from build123d import *

# Parameters (mm, degrees)
F0_W     = 69.0372
F0_H     = 63.5
F1_DEPTH = 4.7625
F2_R     = 3.1877
F3_DEPTH = 4.7635
F4_R     = 2.54
F5_DEPTH = 4.7635
F4_R_2   = 7.527211353
F4_R_3   = 7.5272138977
F6_DEPTH = 0.508
F8_DEPTH = 69.0382


with BuildPart() as f1:
    # F0 (on Top) → F1 (new body)
    with BuildSketch(Plane.XY):
        with Locations((0, -31.75)):
            Rectangle(F0_W, F0_H)
    extrude(amount=F1_DEPTH)

    # F2 (on face) → F3 (cut, through all)
    with BuildSketch(Plane.XY.offset(4.7625)):
        with Locations((25.4, -53.975)):
            Circle(F2_R)
        with Locations((-25.4, -53.975)):
            Circle(F2_R)
    extrude(amount=-F3_DEPTH, mode=Mode.SUBTRACT)

    # F4 (on face) → F5 (cut, through all)
    with BuildSketch(Plane.XY.offset(4.7625)):
        with Locations((-19.05, -19.05)):
            Circle(F4_R)
        with Locations((19.05, -19.05)):
            Circle(F4_R)
    extrude(amount=-F5_DEPTH, mode=Mode.SUBTRACT)

    # F4 (on face) → F6 (cut)
    with BuildSketch(Plane.XY.offset(4.7625)):
        with Locations((-19.05, -19.05)):
            Circle(F4_R_2)
        with Locations((-19.05, -19.05)):
            Circle(F4_R, mode=Mode.SUBTRACT)
        with Locations((19.05, -19.05)):
            Circle(F4_R_3)
        with Locations((19.05, -19.05)):
            Circle(F4_R, mode=Mode.SUBTRACT)
    extrude(amount=-F6_DEPTH, mode=Mode.SUBTRACT)

    # F7 (on face) → F8 (cut, through all)
    with BuildSketch(Plane.YZ.offset(34.5186)):
        with BuildLine():
            ThreePointArc((-1.9939, 4.7625), (-1.5875, 4.3561), (-1.1811, 4.7625))
            Line((-1.1811, 4.7625), (-1.9939, 4.7625))
        make_face()
        with BuildLine():
            Line((-1.9939, 0), (-1.1811, 0))
            ThreePointArc((-1.1811, 0), (-1.5875, 0.4064), (-1.9939, 0))
        make_face()
    extrude(amount=-F8_DEPTH, mode=Mode.SUBTRACT)


solid = f1.part
Work out the finished part from the listing and answer in its coordinate system (mm). A direction names the side the tool comes from. Give positions to 0.01 mm unless a question says otherwise; leave off trailing zeros. Order: outer loops, then holes, each group sorted by start corner. A loop starts at its lowest first (then second) coordinate and runs counter-clockwise, first axis right, second up. Notation, with made-up numbers: (-25, 63.5) -> (7, 63.5) arc R35 cw to (7, 101.5) -> close; hole circle Ø2 at (31, -25). An arc over 180 degrees is marked (long way). One line per item, written item: value.
Item 1: Find section D-D, the plane x = 15. Give the vertices of the cut face in (y, z).
Answer sheet:
outline: (-63.5, 0) -> (-1.99, 0) arc R0.41 cw to (-1.18, 0) -> (0, 0) -> (0, 4.76) -> (-1.18, 4.76) arc R0.41 cw to (-1.99, 4.76) -> (-12.71, 4.76) -> (-12.71, 4.25) -> (-25.39, 4.25) -> (-25.39, 4.76) -> (-63.5, 4.76) -> close
Item 2: Find section A-A, the plane y = -19.05. Give the vertices of the cut face in (x, z).
Answer sheet:
outline: (-34.52, 0) -> (-21.59, 0) -> (-21.59, 4.25) -> (-26.58, 4.25) -> (-26.58, 4.76) -> (-34.52, 4.76) -> close; (-16.51, 0) -> (16.51, 0) -> (16.51, 4.25) -> (11.52, 4.25) -> (11.52, 4.76) -> (-11.52, 4.76) -> (-11.52, 4.25) -> (-16.51, 4.25) -> close; (21.59, 0) -> (34.52, 0) -> (34.52, 4.76) -> (26.58, 4.76) -> (26.58, 4.25) -> (21.59, 4.25) -> close
Item 3: A flat-ended cylindrical pin translates along its axis: P1, Ø7.5, axis at x = 17.5, y = -17, coming from the +Z side. Find the tip coordinate at first contact, or state that the pin passes through.
Answer sheet:
P1: z = 4.25
Item 4: Find section B-B, the plane x = -25.4. Give the vertices of the cut face in (y, z).
Answer sheet:
outline: (-63.5, 0) -> (-57.16, 0) -> (-57.16, 4.76) -> (-63.5, 4.76) -> close; (-50.79, 0) -> (-1.99, 0) arc R0.41 cw to (-1.18, 0) -> (0, 0) -> (0, 4.76) -> (-1.18, 4.76) arc R0.41 cw to (-1.99, 4.76) -> (-15.01, 4.76) -> (-15.01, 4.25) -> (-23.09, 4.25) -> (-23.09, 4.76) -> (-50.79, 4.76) -> close
Item 5: Find section C-C, the plane z = 1.5. Give the vertices of the cut face in (x, y) (3 decimals).
Answer sheet:
outline: (-34.519, -63.5) -> (34.519, -63.5) -> (34.519, 0) -> (-34.519, 0) -> close; hole circle Ø6.375 at (-25.4, -53.975); hole circle Ø5.08 at (-19.05, -19.05); hole circle Ø5.08 at (19.05, -19.05); hole circle Ø6.375 at (25.4, -53.975)
Item 6: Determine the mould class of faces 3 (the flat face through (0, -32, 0)), 4 (the flat face through (0, -63.5, 2)), 5 (the cylindrical face through (26.23, -16.79, 4.51)), 6 (the cylindrical face through (-27.75, -51.82, 2.41)) for opening direction Y: released by +Y, released by -Y, zero draft, split by the parting line, or undercut.
Answer sheet:
face 3: zero draft
face 4: released by -Y
face 5: undercut
face 6: undercut
Item 7: Straight lines are drawn through the part: probe 1 along X at (y, z) = (-55, 2.55); probe 2 along Y at (x, z) = (-17, 0.35); probe 3 along Y at (x, z) = (-19.05, 4.6) (3 decimals). For each, find the intervals that lie inside material, in ascending order.
Answer sheet:
probe 1: -34.52 to -28.42, -22.38 to 22.38, 28.42 to 34.52
probe 2: -63.5 to -20.55, -17.55 to -1.79, -1.38 to 0
probe 3: -63.5 to -26.577, -11.523 to -1.96, -1.215 to 0
Item 8: A tool of negligible diameter and unlimited length cuts with its end or side. For faces 1 (the flat face through (0, -32, 4.762)), 2 (the flat face through (-19, -22, 4.254)), from which of +Z, -Z, +X, -X, +Y, -Y can it reach the whole face along a straight path? Write none if from no direction.
Answer sheet:
face 1: +Z, +X, -X, +Y, -Y
face 2: +Z
